Geometry check sheet. Reference: the model listing, model coordinates, mm. A direction names the side the tool comes from. Round coordinates to 2 decimals unless told otherwise and drop trailing zeros. Write each loop counter-clockwise with the first axis right and the second up, starting at its lowest first coordinate (ties: lowest second). Pieces come first, ordered by that corner, then holes. Notation, with made-up numbers: (39.5, -18.5) -> (89.5, -18.5) arc R14 cw to (89.5, -7.5) -> close; hole circle Ø2 at (65.25, 82.25). An arc over 180 degrees is marked (long way). One line per question, with ' | ' between items.
```python
from build123d import *

# Parameters (mm, degrees)
EXTRUDE_1_DEPTH     = 1
CUT_EXTRUDE_1_DEPTH = 52.40107317
CUT_EXTRUDE_2_DEPTH = 10


with BuildPart() as part:
    # 草图1 → 凸台-拉伸1 (new body)
    with BuildSketch(Plane.XY):
        Polygon((-32, 0), (32, 0), (8.783121635, 40.212812921), (0, 25), (-8.783121635, 40.212812921), align=None)
    extrude(amount=EXTRUDE_1_DEPTH)

    # 草图2 → 切除-拉伸1 (cut, through all)
    with BuildSketch(Plane.XY.offset(1)):
        Polygon((-8.783121635, 25), (-10.515172443, 22), (-8.783121635, 22), align=None)
        Polygon((-11.283121635, 17.669872981), (-11.283121635, 20.669872981), (-13.015172443, 17.669872981), align=None)
        Polygon((-13.783121635, 13.339745962), (-13.783121635, 16.339745962), (-15.515172443, 13.339745962), align=None)
        Polygon((-16.283121635, 9.009618943), (-16.283121635, 12.009618943), (-18.015172443, 9.009618943), align=None)
        Polygon((-18.783121635, 4.679491924), (-18.783121635, 7.679491924), (-20.515172443, 4.679491924), align=None)
        Polygon((-21.283121635, 0.349364905), (-21.283121635, 3.349364905), (-23.015172443, 0.349364905), align=None)
        Polygon((23.015172443, 0.349364905), (21.283121635, 0.349364905), (21.283121635, 3.349364905), align=None)
        Polygon((20.515172443, 4.679491924), (18.783121635, 4.679491924), (18.783121635, 7.679491924), align=None)
        Polygon((18.015172443, 9.009618943), (16.283121635, 9.009618943), (16.283121635, 12.009618943), align=None)
        Polygon((15.515172443, 13.339745962), (13.783121635, 13.339745962), (13.783121635, 16.339745962), align=None)
        Polygon((13.015172443, 17.669872981), (11.283121635, 17.669872981), (11.283121635, 20.669872981), align=None)
        Polygon((10.515172443, 22), (8.783121635, 22), (8.783121635, 25), align=None)
    extrude(amount=-CUT_EXTRUDE_1_DEPTH, mode=Mode.SUBTRACT)

    # 草图3 → 切除-拉伸2 (cut)
    with BuildSketch(Plane.XY.offset(1)):
        Polygon((-11.785343035, 0), (0, 20.412812921), (11.785343035, 0), align=None)
    extrude(amount=-CUT_EXTRUDE_2_DEPTH, mode=Mode.SUBTRACT)


solid = part.part
```
(1) Sectioned sample at C-C on x = -9.5. Record the cut outline in (y, z), then the cut area to 3 significant figures.
Resolved:
outline: (3.96, 0) -> (22, 0) -> (22, 1) -> (3.96, 1) -> close; (23.76, 0) -> (38.97, 0) -> (38.97, 1) -> (23.76, 1) -> close | area: 33.3 mm2
(2) Sectioned sample at B-B on y = 17. Record the cut outline in (x, z), then the cut area to 3 significant figures.
Resolved:
outline: (-22.19, 0) -> (-1.97, 0) -> (-1.97, 1) -> (-22.19, 1) -> close; (1.97, 0) -> (22.19, 0) -> (22.19, 1) -> (1.97, 1) -> close | area: 40.4 mm2
(3) Material ranges on line 1 (X direction, y = 15, z = 0.25); line 2 (X direction, y = 18.5, z = 0.95); line 3 (X direction, y = 38.5, z = 0.8), recorded low to high.
Resolved:
line 1: x = -23.34 to -14.56, -13.78 to -3.13, 3.13 to 13.78, 14.56 to 23.34 | line 2: x = -21.32 to -12.54, -11.28 to -1.1, 1.1 to 11.28, 12.54 to 21.32 | line 3: x = -9.77 to -7.79, 7.79 to 9.77
(4) Access from +Z, -Z, +X, -X, +Y, -Y to the whole of each face (thin tool, end or side, straight path). Record for faces 1 (the flat face through (-4.33, 32.5, 0.49)), 2 (the flat face through (-0.4, 20.4, 0)), 3 (the flat face through (-5.975, 10.064, 0.507)).
Resolved:
face 1: +Z, -Z, +Y | face 2: -Z, +X, -X, +Y, -Y | face 3: +Z, -Z, -Y
(5) Draft check along X on faces 4 (the flat face through (-20.23, 20.39, 0.49)), 5 (the flat face through (19.637, 6.2, 0.507)), 6 (the flat face through (-17.137, 10.531, 0.507)), 7 (the flat face through (20.554, 19.825, 0.493)). Enter one of: +X half, -X half, draft (parallel to the pull), parting line (faces both ways), or undercut.
Resolved:
face 4: -X half | face 5: undercut | face 6: undercut | face 7: +X half
(6) Sectioned sample at D-D on z = 0.45. Count the separate pieces of the cut face and the enclosed holes in it, then the cut area to 3 significant figures.
Resolved:
separate pieces: 1 | enclosed holes: 12 | area: 1,230 mm2
(7) Sectioned sample at A-A on y = 6. Record the cut outline in (x, z), then the cut area to 3 significant figures.
Resolved:
outline: (-28.54, 0) -> (-19.75, 0) -> (-19.75, 1) -> (-28.54, 1) -> close; (-18.78, 0) -> (-8.32, 0) -> (-8.32, 1) -> (-18.78, 1) -> close; (8.32, 0) -> (18.78, 0) -> (18.78, 1) -> (8.32, 1) -> close; (19.75, 0) -> (28.54, 0) -> (28.54, 1) -> (19.75, 1) -> close | area: 38.5 mm2
(8) Go/stop test with flat-tipped pins: pin 1 (0.5 mm diameter, centred on x = 20, z = 0.5, fed in from +Y); pin 2 (0.5 mm diameter, centred on y = 11, z = 0.5, fed in from +X); pin 3 (0.5 mm diameter, centred on y = 15, z = 0.5, fed in from -X). Record where each tip stops, or that it passes through.
Resolved:
pin 1: stops at y = 21.22 | pin 2: stops at x = 25.79 | pin 3: stops at x = -23.48
